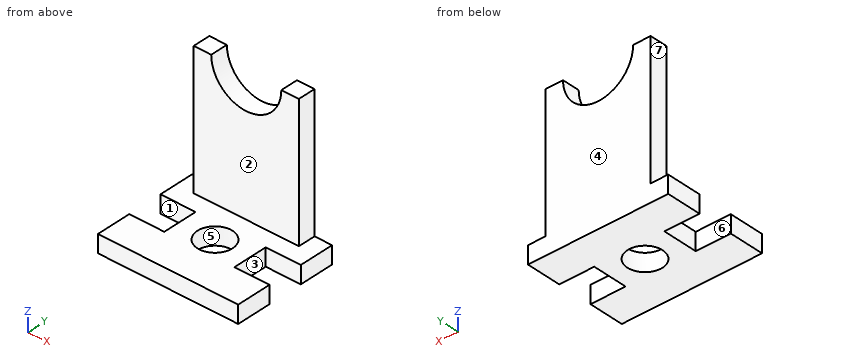
Autodesk Fusion 360 part; units mm, degrees
sketch "Sketch15" plane through (0, 0, 0) normal (0, 0, 1) x (1, 0, 0)
  line L0 (0, 0) -> (200, 0)
  line L1 (200, 0) -> (200, 150)
  line L2 (200, 150) -> (0, 150)
  line L3 (0, 150) -> (0, 0)
  dimension "d98" = 200
  dimension "d99" = 150
extrude "Extrude13" add sketch "Sketch15" along normal blind 25
sketch "Sketch16" plane through (0, 0, 25) normal (0, 0, 1) x (-1, 0, 0)
  line L0 (0, -150) -> (0, 0)
  line L1 (0, 0) -> (-200, 0)
  line L2 (-200, 0) -> (-200, -150)
  line L3 (-200, -150) -> (0, -150)
  line L4 (-200, -50) -> (-150, -50)
  line L5 (-150, -50) -> (-150, -100)
  line L6 (-150, -100) -> (-200, -100)
  line L7 (0, -100) -> (-50, -100)
  line L8 (-50, -100) -> (-50, -50)
  line L9 (-50, -50) -> (0, -50)
  line L10 (0, -75) -> (-100, -75) construction
  circle A0 centre (-100, -75) radius 25
  line L11 (-175, -150) -> (-175, -125)
  line L12 (-175, -125) -> (-25, -125)
  line L13 (-25, -125) -> (-25, -150)
  dimension "d103" = 50
  dimension "d104" = 50
  dimension "d105" = 50
  dimension "d106" = 50
  dimension "d107" = 50
  dimension "d108" = 100
  dimension "d109" = 50
  dimension "d111" = 25
  dimension "d112" = 150
extrude "Extrude14" cut sketch "Sketch16" against normal blind 25 contours L0 L7 L8 L9 | L2 L4 L5 L6
extrude "Extrude15" cut sketch "Sketch16" against normal blind 25 contours A0
extrude "Extrude16" add sketch "Sketch16" along normal blind 190 contours L3 L11 L12 L13
sketch "Sketch17" plane through (0, 125, 0) normal (0, -1, 0) x (1, 0, 0)
  line L0 (25, 25) -> (175, 25)
  line L1 (175, 25) -> (175, 215)
  line L2 (175, 215) -> (25, 215)
  line L3 (25, 215) -> (25, 25)
  line L4 (25, 215) -> (50, 215) construction
  line L5 (175, 215) -> (150, 215) construction
  arc A0 (50, 215) -> (150, 215) centre (100, 215) ccw
  dimension "d119" = 25
  dimension "d120" = 25
  dimension "d121" = 100
extrude "Extrude17" cut sketch "Sketch17" against normal blind 25 contours L2 A0
For this review, take the finished solid that the model builds, in its own axes (mm). Face numbers are marked on the shaded views. A direction names the side the tool comes from. Coordinates: 2 decimals unless noted, no trailing zeros. Order: outer loops, then holes, each group sorted by start corner. A loop starts at its lowest first (then second) coordinate and runs counter-clockwise, first axis right, second up. Notation, with made-up numbers: (86, -7) -> (145, -7) arc R26 ccw to (145, 13) -> close; hole circle Ø6 at (26.25, -21.75). An arc over 180 degrees is marked (long way). Return JSON: item names as keys, results as strings.
1. Machinability: for the marked faces 1, 2, 3 and 4, which of the approach directions +Z, -Z, +X, -X, +Y, -Y give a long, thin tool a straight path to every point of the face, cutting with its end or side? Answer none if there is none.
Answer block:
{"face 1": "+Z, -Z, -X", "face 2": "+Z, +X, -X, -Y", "face 3": "+Z, -Z, +X", "face 4": "+Z, -Z, +X, -X, +Y"}
2. The part is to be moulded in two halves that separate along X. For the marked faces 5, 6 and 7, say which applies: +X half, -X half, draft (parallel to the pull), parting line (faces both ways), or undercut.
Answer block:
{"face 5": "undercut", "face 6": "draft", "face 7": "-X half"}
3. We need section C-C on z = 14.5. Write out the cut boundary in (x, y).
Answer block:
{"outline": "(0, 0) -> (200, 0) -> (200, 50) -> (150, 50) -> (150, 100) -> (200, 100) -> (200, 150) -> (0, 150) -> (0, 100) -> (50, 100) -> (50, 50) -> (0, 50) -> close; hole circle Ø50 at (100, 75)"}
4. For line 1 (Y direction, x = 100, z = 6); line 2 (X direction, y = 75, z = 5); line 3 (Z direction, x = 77.5, y = 98.5), list the stretches that pass through material, from the lowest coordinate up. Write a range as from..to.
Answer block:
{"line 1": "0..50, 100..150", "line 2": "50..75, 125..150", "line 3": "0..25"}
5. We need section A-A on x = 29. Write out the cut boundary in (y, z).
Answer block:
{"outline": "(0, 0) -> (50, 0) -> (50, 25) -> (0, 25) -> close; (100, 0) -> (150, 0) -> (150, 215) -> (125, 215) -> (125, 25) -> (100, 25) -> close"}
6. We need section B-B on y = 75. Write out the cut boundary in (x, z), and give its area (3 significant figures).
Answer block:
{"outline": "(50, 0) -> (75, 0) -> (75, 25) -> (50, 25) -> close; (125, 0) -> (150, 0) -> (150, 25) -> (125, 25) -> close", "area": "1,250 mm²"}
7. For pin 1 Ø8 at (x, y) = (128, 26) entering from +Z; pin 2 Ø20 at (y, z) = (140.5, 99) entering from +X; pin 3 Ø7.5 at (y, z) = (136.5, 114) entering from -X, all flat-tipped, find the tip position at first contact; note any pin that passes through.
Answer block:
{"pin 1": "z = 25", "pin 2": "x = 175", "pin 3": "x = 25"}
8. We need section D-D on z = 170.5. Write out the cut boundary in (x, y).
Answer block:
{"outline": "(25, 125) -> (77.2, 125) -> (77.2, 150) -> (25, 150) -> close; (122.8, 125) -> (175, 125) -> (175, 150) -> (122.8, 150) -> close"}
